from build123d import *

# Parameters (mm, degrees)
CROQUIS1_W                       = 94
CROQUIS1_H                       = 192
BRIDA_BASE1_DEPTH                = 1.5
BRIDA_DE_ARISTA1_STRIP_CUT_DEPTH = 192
BRIDA_DE_ARISTA1_DEPTH           = 192
BRIDA_DE_ARISTA3_STRIP_CUT_DEPTH = 192
BRIDA_DE_ARISTA3_DEPTH           = 192
BRIDA_DE_ARISTA4_STRIP_W         = 7.4732
BRIDA_DE_ARISTA4_STRIP_H         = 1.5
BRIDA_DE_ARISTA4_STRIP_CUT_DEPTH = 192
BRIDA_DE_ARISTA4_DEPTH           = 192
DOBLADILLO1_START                = -96
DOBLADILLO1_DEPTH                = 192
DOBLADILLO1_2_DEPTH              = 192


# Read off the part's stored shape, not the designer's step: Dobladillo1
# Sheet-metal steps are written as plain solids
with BuildPart() as part:
    # Croquis1 → Brida base1 (new body)
    with BuildSketch(Plane(origin=(0, 0, 0), x_dir=(1, 0, 0), z_dir=(0, 1, 0))):
        Rectangle(CROQUIS1_W, CROQUIS1_H)
    extrude(amount=BRIDA_BASE1_DEPTH)

    # Brida de arista1 strip (across the edge) → Brida de arista1 strip cut (cut)
    with BuildSketch(Plane(origin=(47, 1.5, 96), x_dir=(-0.7071067811865438, 0.7071067811865512, 0), z_dir=(0, 0, -1))):
        Polygon((-6.129265424, 4.00794508), (-0.844915027, -1.276405317), (0.215745145, -0.215745145), (-5.068605252, 5.068605252), align=None)
    extrude(amount=BRIDA_DE_ARISTA1_STRIP_CUT_DEPTH, mode=Mode.SUBTRACT)

    # Brida de arista1 section (across the edge) → Brida de arista1 (add)
    with BuildSketch(Plane(origin=(47, 1.5, 96), x_dir=(-0.7071067811865438, 0.7071067811865512, 0), z_dir=(0, 0, -1))):
        with BuildLine():
            Line((-1.5, 0.30510971), (-1.5, 23.420310217))
            Line((-1.5, 23.420310217), (0, 23.420310217))
            Line((0, 23.420310217), (0, 0.30510971))
            ThreePointArc((0, 0.30510971), (0.056070336, 0.023225094), (0.215745145, -0.215745145))
            Line((0.215745145, -0.215745145), (-0.844915027, -1.276405317))
            ThreePointArc((-0.844915027, -1.276405317), (-1.329748962, -0.550800055), (-1.5, 0.30510971))
        make_face()
    extrude(amount=BRIDA_DE_ARISTA1_DEPTH)

    # Brida de arista3 strip (across the edge) → Brida de arista3 strip cut (cut)
    with BuildSketch(Plane(origin=(63.560660172, 18.060660172, 96), x_dir=(-1, 0, 0), z_dir=(0, 0, -1))):
        Polygon((-6.129265424, 4.00794508), (-0.844915027, -1.276405317), (0.215745145, -0.215745145), (-5.068605252, 5.068605252), align=None)
    extrude(amount=BRIDA_DE_ARISTA3_STRIP_CUT_DEPTH, mode=Mode.SUBTRACT)

    # Brida de arista3 section (across the edge) → Brida de arista3 (add)
    with BuildSketch(Plane(origin=(63.560660172, 18.060660172, 96), x_dir=(-1, 0, 0), z_dir=(0, 0, -1))):
        with BuildLine():
            Line((-1.5, 0.30510971), (-1.5, 94.978679656))
            Line((-1.5, 94.978679656), (0, 94.978679656))
            Line((0, 94.978679656), (0, 0.30510971))
            ThreePointArc((0, 0.30510971), (0.056070336, 0.023225094), (0.215745145, -0.215745145))
            Line((0.215745145, -0.215745145), (-0.844915027, -1.276405317))
            ThreePointArc((-0.844915027, -1.276405317), (-1.329748962, -0.550800055), (-1.5, 0.30510971))
        make_face()
    extrude(amount=BRIDA_DE_ARISTA3_DEPTH)

    # Brida de arista4 strip (across the edge) → Brida de arista4 strip cut (cut)
    with BuildSketch(Plane(origin=(63.560660172, 113.039339828, 96), x_dir=(0, -1, 0), z_dir=(0, 0, -1))):
        with Locations((-1.5, -0.75)):
            Rectangle(BRIDA_DE_ARISTA4_STRIP_W, BRIDA_DE_ARISTA4_STRIP_H)
    extrude(amount=BRIDA_DE_ARISTA4_STRIP_CUT_DEPTH, mode=Mode.SUBTRACT)

    # Brida de arista4 section (across the edge) → Brida de arista4 (add)
    with BuildSketch(Plane(origin=(63.560660172, 113.039339828, 96), x_dir=(0, -1, 0), z_dir=(0, 0, -1))):
        with BuildLine():
            Line((0, 0.7366), (0, 18))
            Line((0, 18), (1.5, 18))
            Line((1.5, 18), (1.5, 0.7366))
            ThreePointArc((1.5, 0.7366), (1.715745145, 0.215745145), (2.2366, 0))
            Line((2.2366, 0), (2.2366, -1.5))
            ThreePointArc((2.2366, -1.5), (0.655084973, -0.844915027), (0, 0.7366))
        make_face()
    extrude(amount=BRIDA_DE_ARISTA4_DEPTH)

    # Dobladillo1 outline → Dobladillo1 (cut)
    with BuildSketch(Plane.XY.offset(DOBLADILLO1_START)):
        with BuildLine():
            Line((45.560660172, 111.539339828), (45.561466834, 111.539339828))
            ThreePointArc((45.561466834, 111.539339828), (46.032467239, 112.602892701), (47.110660172, 113.039339828))
            Line((47.110660172, 113.039339828), (45.560660172, 113.039339828))
            Line((45.560660172, 113.039339828), (45.560660172, 111.539339828))
        make_face()
        with BuildLine():
            ThreePointArc((-45.45, 0), (-46.528192933, 0.436447127), (-46.999193338, 1.5))
            Line((-46.999193338, 1.5), (-47, 1.5))
            Line((-47, 1.5), (-47, 0))
            Line((-47, 0), (-45.45, 0))
        make_face()
    extrude(amount=DOBLADILLO1_DEPTH, mode=Mode.SUBTRACT)

    # Dobladillo1 2 outline → Dobladillo1 2 (add)
    with BuildSketch(Plane.XY.offset(DOBLADILLO1_START)):
        with BuildLine():
            Line((54.060660172, 109.939339828), (54.060660172, 111.439339828))
            Line((54.060660172, 111.439339828), (47.110660172, 111.439339828))
            ThreePointArc((47.110660172, 111.439339828), (47.060660172, 111.489339828), (47.110660172, 111.539339828))
            Line((47.110660172, 111.539339828), (45.561466834, 111.539339828))
            ThreePointArc((45.561466834, 111.539339828), (45.997107299, 110.411146895), (47.110660172, 109.939339828))
            Line((47.110660172, 109.939339828), (54.060660172, 109.939339828))
        make_face()
        with BuildLine():
            Line((-38.5, 1.6), (-38.5, 3.1))
            Line((-38.5, 3.1), (-45.45, 3.1))
            ThreePointArc((-45.45, 3.1), (-46.563552873, 2.628192933), (-46.999193338, 1.5))
            Line((-46.999193338, 1.5), (-45.45, 1.5))
            ThreePointArc((-45.45, 1.5), (-45.5, 1.55), (-45.45, 1.6))
            Line((-45.45, 1.6), (-38.5, 1.6))
        make_face()
    extrude(amount=DOBLADILLO1_2_DEPTH)


solid = part.part
Verification items for the finished model (mm, model axes). A direction names the side the tool comes from. Round coordinates to 2 decimals unless told otherwise and drop trailing zeros. Loops run counter-clockwise (first coordinate to the right, second up) from the corner with the lowest first, then second, coordinate; pieces in that order, holes last. Notation, with made-up numbers: M 81.25,-19 L 109.25,-19 A29 ccw 109.25,11 Z; hole C 61,88.5 d6. An arc over 180 degrees is marked long. Write each question's results on one line, items separated by ' | '.
1) Access from +Z, -Z, +X, -X, +Y, -Y to the whole of each face (thin tool, end or side, straight path). Record for faces 1 (the flat face through (-42, 3.1, -1)), 2 (the flat face through (0, 0, -1)).
Checks:
face 1: +Z, -Z, -X, +Y | face 2: +Z, -Z, +X, -X, -Y
2) Gauge pin test, flat ends, axial feed: P1, Ø5.5, axis at x = -42.5, z = -29.5, coming from the +Y side; P2, Ø8, axis at x = 52, z = 29.5, coming from the -Y side; P3, Ø12, axis at y = 43.5, z = 61.5, coming from the -X side. Record the tip position at first contact, or that the pin passes through.
Checks:
P1: stops at y = 3.1 | P2: stops at y = 0.42 | P3: stops at x = 63.56
3) Scan lines: L1, parallel to Y at x = 35, z = -4.5; L2, parallel to X at y = 27.5, z = 6; L3, parallel to Y at x = 56, z = 55. Record each from-to range of solid material in increasing order. Write a range as from..to.
Checks:
L1: y = 0..1.5 | L2: x = 63.56..65.06 | L3: y = 8.38..10.5, 111.54..113.04
4) Section check A-A on z = 44.5. Record the boundary of the cut face in (x, y).
Checks:
outline: M -45.45,0 L 46.69,0 A2.24 ccw 48.28,0.66 L 64.41,16.78 A2.24 ccw 65.06,18.37 L 65.06,110.8 A2.24 ccw 62.82,113.04 L 47.11,113.04 A1.55 ccw 47.11,109.94 L 54.06,109.94 L 54.06,111.44 L 47.11,111.44 A0.05 cw 47.11,111.54 L 62.82,111.54 A0.74 cw 63.56,110.8 L 63.56,18.37 A0.74 cw 63.34,17.84 L 47.22,1.72 A0.74 cw 46.69,1.5 L -45.45,1.5 A0.05 cw -45.45,1.6 L -38.5,1.6 L -38.5,3.1 L -45.45,3.1 A1.55 ccw Z
5) Section check C-C on y = 78.5. Record the boundary of the cut face in (x, z), then the cut area to 3 significant figures.
Checks:
outline: M 63.56,-96 L 65.06,-96 L 65.06,96 L 63.56,96 Z | area: 288 mm2
6) Mould release check, pull along X, two halves, no side actions. Record for faces 3 (the flat face through (56.23, 8.61, 1.34)), 4 (the flat face through (55, 111.539, 1)), 5 (the flat face through (51, 109.939, -1)), 6 (the flat face through (0, 1.5, -1)): released by +X, released by -X, zero draft, split by the parting line, or undercut.
Checks:
face 3: released by +X | face 4: undercut | face 5: zero draft | face 6: undercut
7) Section check B-B on x = 0. Record the boundary of the cut face in (y, z).
Checks:
outline: M 0,-96 L 1.5,-96 L 1.5,96 L 0,96 Z
